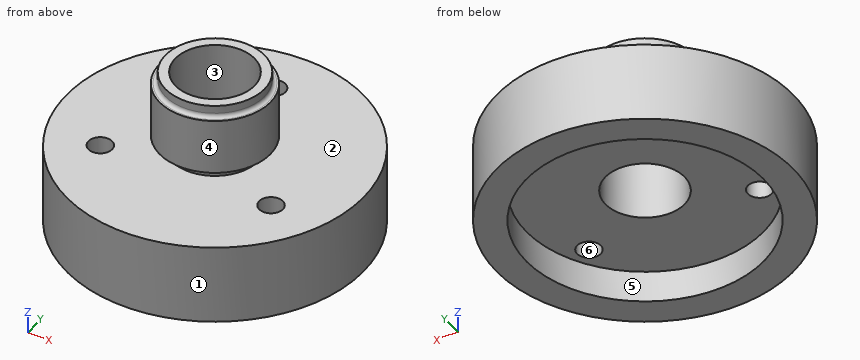
from build123d import *

# Parameters (mm, degrees)
SKETCH004_R        = 24.41662
SKETCH004_R_2      = 11
PAD002_DEPTH       = 3
SKETCH_R           = 37.5
PAD_DEPTH          = 20
SKETCH001_R        = 30
POCKET_DEPTH       = 8
SKETCH002_R        = 3
POCKET001_DEPTH    = 235.871331
POLARPATTERN_COUNT = 3
SKETCH003_R        = 14
PAD001_DEPTH       = 20
SKETCH005_R        = 10
POCKET002_DEPTH    = 40.001
SKETCH006_R        = 20.656229
SKETCH006_R_2      = 12.5
POCKET003_DEPTH    = 3
FILLET_R           = 1
FILLET001_R        = 1


with BuildPart() as pad002:
    # Sketch004 → Pad002 (new body)
    with BuildSketch(Plane.XY.offset(20)):
        Circle(SKETCH004_R)
        Circle(SKETCH004_R_2, mode=Mode.SUBTRACT)
    extrude(amount=PAD002_DEPTH)


with BuildPart() as fillet001:
    # Sketch → Pad (new body)
    with BuildSketch(Plane.XY):
        Circle(SKETCH_R)
    extrude(amount=PAD_DEPTH)

    # Sketch001 → Pocket (cut)
    with BuildSketch(Plane(origin=(0, 0, 0), x_dir=(1, 0, 0), z_dir=(0, 0, -1))):
        Circle(SKETCH001_R)
    extrude(amount=-POCKET_DEPTH, mode=Mode.SUBTRACT)

    # Sketch002 → Pocket001 (cut, through all)
    with BuildSketch(Plane.XY.offset(20)):
        with Locations((0, 25)):
            Circle(SKETCH002_R)
    pocket001 = extrude(amount=-POCKET001_DEPTH, mode=Mode.SUBTRACT)

    # PolarPattern: Pocket001 ×3 about axis
    polarpattern_axis = Axis((0, 0, 20), (0, 0, 1))
    for i in range(1, POLARPATTERN_COUNT):
        add(pocket001.rotate(polarpattern_axis, i * 360 / POLARPATTERN_COUNT), mode=Mode.SUBTRACT)

    # Sketch003 → Pad001 (new body)
    with BuildSketch(Plane.XY.offset(20)):
        Circle(SKETCH003_R)
    extrude(amount=PAD001_DEPTH)

    # Cut: cut Pad002
    add(pad002.part, mode=Mode.SUBTRACT)

    # Sketch005 → Pocket002 (cut, through all)
    with BuildSketch(Plane.XY.offset(40)):
        Circle(SKETCH005_R)
    extrude(amount=-POCKET002_DEPTH, mode=Mode.SUBTRACT)

    # Sketch006 → Pocket003 (cut)
    with BuildSketch(Plane.XY.offset(40)):
        Circle(SKETCH006_R)
        Circle(SKETCH006_R_2, mode=Mode.SUBTRACT)
    extrude(amount=-POCKET003_DEPTH, mode=Mode.SUBTRACT)

    # Fillet
    fillet_edges = [fillet001.edges().sort_by_distance(p)[0] for p in [
        (-12.5, 0, 37),
    ]]
    fillet(fillet_edges, radius=FILLET_R)

    # Fillet001
    fillet001_edges = [fillet001.edges().sort_by_distance(p)[0] for p in [
        (-11, 0, 23),
    ]]
    fillet(fillet001_edges, radius=FILLET001_R)


solid = fillet001.part
Geometry check sheet. Reference: the model listing, model coordinates, mm. Face numbers are marked on the shaded views. A direction names the side the tool comes from. Give positions to 0.01 mm unless a question says otherwise; leave off trailing zeros. Loops run counter-clockwise (first coordinate to the right, second up) from the corner with the lowest first, then second, coordinate; pieces in that order, holes last. Notation, with made-up numbers: M -8.5,72 L 20.5,72 A19 ccw 20.5,83 Z; hole C 60.25,1 d8. An arc over 180 degrees is marked long. Answer as a JSON object with one key per item and string values. Group by question number.
Item 1: Gauge pin test, flat ends, axial feed: pin 1 (1.5 mm diameter, centred on x = 19, y = 20, fed in from +Z); pin 2 (22.5 mm diameter, centred on x = 6, y = 4, fed in from -Z); pin 3 (1.5 mm diameter, centred on x = -3, z = 19.5, fed in from +Y); pin 4 (14 mm diameter, centred on x = 2, y = 2, fed in from +Z). Record the tip position at first contact, or that the pin passes through.
Item 2: Sectioned sample at B-B on x = 0. Give the number of separate pieces and of enclosed holes in the cut face, plus the area to 3 significant figures.
Item 3: Sectioned sample at D-D on z = 28. Record the boundary of the cut face in (x, y).
Item 4: Material ranges on L1, parallel to Y at x = 0, z = 16.25; L2, parallel to X at y = -1, z = 6.5; L3, parallel to Z at x = 24.5, y = 0.5, recorded low to high.
Item 5: Sectioned sample at A-A on y = 0. Record the boundary of the cut face in (x, z), plus the area to 3 significant figures.
Item 6: Mould release check, pull along X, two halves, no side actions. Record for the marked faces 1, 2 and 3: pulls with the +X half, pulls with the -X half, needs draft (parallel to the pull), parting line crosses it, or undercut.
Item 7: Sectioned sample at C-C on x = 22. Record the boundary of the cut face in (y, z).
Item 8: Access from +Z, -Z, +X, -X, +Y, -Y to the whole of each face (thin tool, end or side, straight path). Record for the marked faces 4, 5 and 6.
Findings below:
{
 "1": {"pin 1": "z = 20", "pin 2": "z = 8", "pin 3": "y = 37.43", "pin 4": "through"},
 "2": {"separate pieces": "3", "enclosed holes": "0", "area": "842 mm2"},
 "3": {"outline": "C 0,0 d28; hole C 0,0 d20"},
 "4": {"L1": "-37.5 to -10, 10 to 22, 28 to 37.5", "L2": "-37.49 to -29.98, 29.98 to 37.49", "L3": "8 to 20"},
 "5": {"outline": "M -37.5,0 L -30,0 L -30,8 L -10,8 L -10,40 L -12.5,40 L -12.5,38 A1 cw -13.5,37 L -14,37 L -14,23 L -12,23 A1 cw -11,22 L -11,20 L -37.5,20 Z; M 10,8 L 30,8 L 30,0 L 37.5,0 L 37.5,20 L 11,20 L 11,22 A1 cw 12,23 L 14,23 L 14,37 L 13.5,37 A1 cw 12.5,38 L 12.5,40 L 10,40 Z", "area": "914 mm2"},
 "6": {"face 1": "parting line crosses it", "face 2": "needs draft", "face 3": "undercut"},
 "7": {"outline": "M -30.37,0 L -20.4,0 L -20.4,8 L -15.48,8 L -15.48,20 L -30.37,20 Z; M -9.52,8 L 20.4,8 L 20.4,0 L 30.37,0 L 30.37,20 L -9.52,20 Z"},
 "8": {"face 4": "+Z", "face 5": "-Z", "face 6": "+Z, -Z"}
}
